from build123d import *

# Parameters (mm, degrees)
BOSS_EXTRUDE1_DEPTH    = 12.7
CUT_EXTRUDE1_DEPTH     = 12.7
CONVERT_SOLID1_DEPTH   = 12.7
CONVERT_SOLID1_2_DEPTH = 12.7


# Read off the part's stored shape, not the designer's step: Convert-Solid1
with BuildPart() as part:
    # Sketch1 → Boss-Extrude1 (new body)
    with BuildSketch(Plane.XY):
        Polygon((0, 0), (10, 0), (17, -7), (51.5, -7), (56, -2.5), (72.5, -2.5), (72.5, -7), (73.77, -7), (73.77, -1.23), (55.473948776, -1.23), (50.973948776, -5.73), (17.526051224, -5.73), (10.526051224, 1.27), (0, 1.27), (-10.526051224, 1.27), (-17.526051224, -5.73), (-50.973948776, -5.73), (-55.473948776, -1.23), (-73.77, -1.23), (-73.77, -7), (-72.5, -7), (-72.5, -2.5), (-56, -2.5), (-51.5, -7), (-17, -7), (-10, 0), align=None)
    extrude(amount=BOSS_EXTRUDE1_DEPTH)

    # Sketch2 → Cut-Extrude1 (cut)
    with BuildSketch(Plane(origin=(0, 1.27, 0), x_dir=(1, 0, 0), z_dir=(0, 1, 0))):
        with BuildLine():
            Line((-2.15, -3.3), (2.15, -3.3))
            ThreePointArc((2.15, -3.3), (2.786396103, -3.563603897), (3.05, -4.2))
            Line((3.05, -4.2), (3.05, -8.5))
            ThreePointArc((3.05, -8.5), (2.786396103, -9.136396103), (2.15, -9.4))
            Line((2.15, -9.4), (-2.15, -9.4))
            ThreePointArc((-2.15, -9.4), (-2.786396103, -9.136396103), (-3.05, -8.5))
            Line((-3.05, -8.5), (-3.05, -4.2))
            ThreePointArc((-3.05, -4.2), (-2.786396103, -3.563603897), (-2.15, -3.3))
        make_face()
    extrude(amount=-CUT_EXTRUDE1_DEPTH, mode=Mode.SUBTRACT)

    # Convert-Solid1 outline → Convert-Solid1 (cut)
    with BuildSketch(Plane.XY):
        with BuildLine():
            Line((73.77, -1.23), (72, -1.23))
            ThreePointArc((72, -1.23), (73.251579003, -1.748420997), (73.77, -3))
            Line((73.77, -3), (73.77, -1.23))
        make_face()
        with BuildLine():
            ThreePointArc((54.955527778, -1.748420997), (55.529757106, -1.364733227), (56.207106781, -1.23))
            Line((56.207106781, -1.23), (55.473948776, -1.23))
            Line((55.473948776, -1.23), (54.955527778, -1.748420997))
        make_face()
        with BuildLine():
            ThreePointArc((9.792893219, 1.27), (10.470242894, 1.135266773), (11.044472222, 0.751579003))
            Line((11.044472222, 0.751579003), (10.526051224, 1.27))
            Line((10.526051224, 1.27), (9.792893219, 1.27))
        make_face()
        with BuildLine():
            Line((51.5, -7), (52.018420997, -6.481579003))
            ThreePointArc((52.018420997, -6.481579003), (51.44419167, -6.865266773), (50.766841995, -7))
            Line((50.766841995, -7), (51.5, -7))
        make_face()
        with BuildLine():
            ThreePointArc((-11.044472222, 0.751579003), (-10.470242894, 1.135266773), (-9.792893219, 1.27))
            Line((-9.792893219, 1.27), (-10.526051224, 1.27))
            Line((-10.526051224, 1.27), (-11.044472222, 0.751579003))
        make_face()
        with BuildLine():
            Line((17, -7), (17.733158005, -7))
            ThreePointArc((17.733158005, -7), (17.05580833, -6.865266773), (16.481579003, -6.481579003))
            Line((16.481579003, -6.481579003), (17, -7))
        make_face()
        with BuildLine():
            ThreePointArc((-56.207106781, -1.23), (-55.529757106, -1.364733227), (-54.955527778, -1.748420997))
            Line((-54.955527778, -1.748420997), (-55.473948776, -1.23))
            Line((-55.473948776, -1.23), (-56.207106781, -1.23))
        make_face()
        with BuildLine():
            Line((-17, -7), (-16.481579003, -6.481579003))
            ThreePointArc((-16.481579003, -6.481579003), (-17.05580833, -6.865266773), (-17.733158005, -7))
            Line((-17.733158005, -7), (-17, -7))
        make_face()
        with BuildLine():
            ThreePointArc((-73.77, -3), (-73.251579003, -1.748420997), (-72, -1.23))
            Line((-72, -1.23), (-73.77, -1.23))
            Line((-73.77, -1.23), (-73.77, -3))
        make_face()
        with BuildLine():
            Line((-51.5, -7), (-50.766841995, -7))
            ThreePointArc((-50.766841995, -7), (-51.44419167, -6.865266773), (-52.018420997, -6.481579003))
            Line((-52.018420997, -6.481579003), (-51.5, -7))
        make_face()
    extrude(amount=CONVERT_SOLID1_DEPTH, mode=Mode.SUBTRACT)

    # Convert-Solid1 2 outline → Convert-Solid1 2 (add)
    with BuildSketch(Plane.XY):
        with BuildLine():
            Line((50.973948776, -5.73), (51.120395385, -5.583553391))
            ThreePointArc((51.120395385, -5.583553391), (50.958183711, -5.691939766), (50.766841995, -5.73))
            Line((50.766841995, -5.73), (50.973948776, -5.73))
        make_face()
        with BuildLine():
            ThreePointArc((72, -2.5), (72.353553391, -2.646446609), (72.5, -3))
            Line((72.5, -3), (72.5, -2.5))
            Line((72.5, -2.5), (72, -2.5))
        make_face()
        with BuildLine():
            Line((17.526051224, -5.73), (17.733158005, -5.73))
            ThreePointArc((17.733158005, -5.73), (17.541816289, -5.691939766), (17.379604615, -5.583553391))
            Line((17.379604615, -5.583553391), (17.526051224, -5.73))
        make_face()
        with BuildLine():
            ThreePointArc((55.853553391, -2.646446609), (56.015765065, -2.538060234), (56.207106781, -2.5))
            Line((56.207106781, -2.5), (56, -2.5))
            Line((56, -2.5), (55.853553391, -2.646446609))
        make_face()
        with BuildLine():
            Line((-17.526051224, -5.73), (-17.379604615, -5.583553391))
            ThreePointArc((-17.379604615, -5.583553391), (-17.541816289, -5.691939766), (-17.733158005, -5.73))
            Line((-17.733158005, -5.73), (-17.526051224, -5.73))
        make_face()
        with BuildLine():
            ThreePointArc((9.792893219, 0), (9.984234935, -0.038060234), (10.146446609, -0.146446609))
            Line((10.146446609, -0.146446609), (10, 0))
            Line((10, 0), (9.792893219, 0))
        make_face()
        with BuildLine():
            Line((-50.973948776, -5.73), (-50.766841995, -5.73))
            ThreePointArc((-50.766841995, -5.73), (-50.958183711, -5.691939766), (-51.120395385, -5.583553391))
            Line((-51.120395385, -5.583553391), (-50.973948776, -5.73))
        make_face()
        with BuildLine():
            ThreePointArc((-10.146446609, -0.146446609), (-9.984234935, -0.038060234), (-9.792893219, 0))
            Line((-9.792893219, 0), (-10, 0))
            Line((-10, 0), (-10.146446609, -0.146446609))
        make_face()
        with BuildLine():
            ThreePointArc((-56.207106781, -2.5), (-56.015765065, -2.538060234), (-55.853553391, -2.646446609))
            Line((-55.853553391, -2.646446609), (-56, -2.5))
            Line((-56, -2.5), (-56.207106781, -2.5))
        make_face()
        with BuildLine():
            Line((-72.5, -2.5), (-72.5, -3))
            ThreePointArc((-72.5, -3), (-72.353553391, -2.646446609), (-72, -2.5))
            Line((-72, -2.5), (-72.5, -2.5))
        make_face()
    extrude(amount=CONVERT_SOLID1_2_DEPTH)


solid = part.part
Check sheet for the modelled part. Datum: model origin and axes. Units: mm. A direction names the side the tool comes from. Give positions to 0.01 mm unless a question says otherwise; leave off trailing zeros. Loops run counter-clockwise (first coordinate to the right, second up) from the corner with the lowest first, then second, coordinate; pieces in that order, holes last. Notation, with made-up numbers: M 17,55 L 72,55 A6 cw 72,60 Z; hole C 34.5,6 d9. An arc over 180 degrees is marked long. Answer as a JSON object with one key per item and string values. Group by question number.
Q1. Cross-section at A-A on x = 31.5. Record the cut outline in (y, z), then the cut area to 3 significant figures.
Q2. Release check for a two-part mould opening along X. For faces 1 (the flat face through (-72.5, -5, 6)), 2 (the flat face through (-73.77, -5, 6)), 3 (the flat face through (-0.3, 0.2, 0)) record: released by +X, released by -X, zero draft, split by the parting line, or undercut.
Q3. Material ranges on line 1 along X through (y, z) = (-4.25, 6.25); line 2 along X through (y, z) = (-5.25, 4.25); line 3 along X through (y, z) = (-6.25, 11), recorded low to high. Write a range as [from, to].
Q4. Cross-section at B-B on x = 15. Record the cut outline in (y, z).
Q5. Go/stop test with flat-tipped pins: P1, Ø3, axis at x = -53, z = 6.5, coming from the +Y side; P2, Ø6.5, axis at x = -37, z = 8, coming from the +Y side; P3, Ø1, axis at x = 0.5, y = 0.5, coming from the -Z side; P4, Ø1.4, axis at y = 0.5, z = 6.5, coming from the +X side. Record where each tip stops, or that it passes through.
Q6. Access from +Z, -Z, +X, -X, +Y, -Y to the whole of each face (thin tool, end or side, straight path). Record for faces 4 (the flat face through (-53.011, -3.693, 6.261)), 5 (the flat face through (-13, -3, 6)), 6 (the flat face through (-34, -7, 6)).
Evaluation:
{
 "1": {"outline": "M -7,0 L -5.73,0 L -5.73,12.7 L -7,12.7 Z", "area": "16.1 mm2"},
 "2": {"face 1": "undercut", "face 2": "released by -X", "face 3": "zero draft"},
 "3": {"line 1": "x = [-73.77, -72.5], [-54.25, -52.45], [-16.05, -14.25], [14.25, 16.05], [52.45, 54.25], [72.5, 73.77]", "line 2": "x = [-73.77, -72.5], [-53.25, -51.45], [-17.05, -15.25], [15.25, 17.05], [51.45, 53.25], [72.5, 73.77]", "line 3": "x = [-73.77, -72.5], [-52.25, -16.25], [16.25, 52.25], [72.5, 73.77]"},
 "4": {"outline": "M -5,0 L -3.2,0 L -3.2,12.7 L -5,12.7 Z"},
 "5": {"P1": "stops at y = -2.2", "P2": "stops at y = -5.73", "P3": "stops at z = 0", "P4": "stops at x = 12"},
 "6": {"face 4": "+Z, -Z, +Y", "face 5": "+Z, -Z, -Y", "face 6": "+Z, -Z, +X, -X, -Y"}
}
